CAD build for the part. Positions are in the model's coordinates, mm. Coordinates: 2 decimals unless noted, no trailing zeros. Write each loop counter-clockwise with the first axis right and the second up, starting at its lowest first coordinate (ties: lowest second). Pieces come first, ordered by that corner, then holes. Notation, with made-up numbers: (2, 42.5) - (55, 42.5) arc R31 cw to (55, 79.5) - close; hole circle Ø8 at (12.25, 66). An arc over 180 degrees is marked (long way). One line per question, with ' | ' between items. Start each with the question number.
1. Probe line 1 (Y direction, x = -5.5, z = -0.3); line 2 (Y direction, x = -2.5, z = 0.25); line 3 (X direction, y = 29.5, z = 0). List the from-to ranges inside material, lowest first.
2. Flat gauge pins, fed straight in: P1, Ø8, axis at x = -5, y = 113.5, coming from the -Z side; P2, Ø5, axis at x = -3, y = 74, coming from the -Z side. Where does each tip first touch, or does it go through?
3. Band-saw the part on A-A, the plane y = 37. Write the cut outline in (x, z) (1 decimal).
from build123d import *
from build123d.topology import SkipClean

# Parameters (mm, degrees)
SKETCH1_R               = 1.5875
BOSS_EXTRUDE1_DEPTH     = 152.4
SKETCH3_R               = 1.5875
DOME1_FACE_RADIUS       = 1.5875
DOME1_HEIGHT            = 6.35
CUT_EXTRUDE1_DEPTH      = 177.879432926
CUT_EXTRUDE1_DEPTH_BACK = 177.879432926
SKETCH5_R               = 0.396875


with BuildPart() as part:
    # Sketch1 → Boss-Extrude1 (new body)
    with BuildSketch(Plane(origin=(0, 0, 0), x_dir=(1, 0, 0), z_dir=(0, 1, 0))):
        with Locations(Location((0, 0, 0), (0, 0, 90))):
            Circle(SKETCH1_R)
    extrude(amount=BOSS_EXTRUDE1_DEPTH)

    # Sweep1: sweep along a path in Sketch2
    with SkipClean():  # the faces are left unmerged after this step: merging them gives an invalid solid
        with BuildLine(Plane.XY) as sweep1_path:
            Line((0, 152.4), (0, 154.94))
            ThreePointArc((0, 154.94), (-0.554390662, 156.523968294), (-1.975555556, 157.416489949))
            ThreePointArc((-1.975555556, 157.416489949), (-0.291800096, 174.969414545), (2.54, 157.564785778))
        # Sketch3 → Sweep1 (sweep)
        with BuildSketch(Plane(origin=(0, 152.4, 0), x_dir=(1, 0, 0), z_dir=(0, 1, 0))):
            Circle(SKETCH3_R)
        sweep(path=sweep1_path.line)

    # Dome1: an elliptical dome of height H over a round flat face of radius A is half a spheroid: the quarter ellipse of half axes A and H revolved about the face's axis
    with BuildSketch(Plane((0, 0, 0), x_dir=(0, 0, 1), z_dir=(1, 0, 0)), mode=Mode.PRIVATE) as dome1_quarter:
        Ellipse(DOME1_FACE_RADIUS, DOME1_HEIGHT)
        Rectangle(DOME1_FACE_RADIUS, DOME1_HEIGHT, align=(Align.MIN, Align.MIN), mode=Mode.INTERSECT)
    revolve(dome1_quarter.sketch, axis=Axis((0, 0, 0), (0, -1, 0)))

    # Sketch5 → Cut-Extrude1 (cut, two sides: drawn at the far end of the back side and taken through both)
    with BuildSketch(Plane(origin=(0, 0, 0), x_dir=(0, 0, -1), z_dir=(1, 0, 0)).offset(-CUT_EXTRUDE1_DEPTH_BACK)):
        with Locations((0, 0.635)):
            Circle(SKETCH5_R)
    extrude(amount=CUT_EXTRUDE1_DEPTH + CUT_EXTRUDE1_DEPTH_BACK, mode=Mode.SUBTRACT)


solid = part.part
Filled in:
1) line 1: y = 157.2 to 161.24, 170.93 to 174.97 | line 2: y = 155.93 to 159.2, 172.97 to 176.24 | line 3: x = -1.59 to 1.59
2) P1: stops at z = -1.23 | P2: stops at z = -1.51
3) outline: circle Ø3.2 at (0, 0)
